Input: part model. Units: mm. Frame: model coordinates. Face numbers are marked on the shaded views. A direction names the side the tool comes from. Round coordinates to 2 decimals unless told otherwise and drop trailing zeros. Order: outer loops, then holes, each group sorted by start corner. A loop starts at its lowest first (then second) coordinate and runs counter-clockwise, first axis right, second up.
Item 1: Reachability of the marked faces 1 and 2 from +Z, -Z, +X, -X, +Y, -Y: full face, straight path, thin tool, end or side. Return the list, or none.
Item 2: Cut plane B-B on x = 7.5. Output: boundary loops of the cut face in (y, z).
Item 3: Cut plane D-D on z = 8. Give the number of separate pieces and of enclosed holes in the cut face, then the cut area to 3 significant figures.
Item 4: Mould query, pull axis X, two halves, no side actions, for the marked faces 3, 4, 5 and 6. Classes: released by +X, released by -X, zero draft, split by the parting line, or undercut.
Item 5: Line query: L1, parallel to X at y = 32, z = 8; L2, parallel to X at y = -19, z = 6; L3, parallel to Y at x = 36, z = 8.25. Output: solid intervals per line, ascending.
Item 6: Cut plane C-C on y = -7.5. Output: boundary loops of the cut face in (x, z).
Item 7: Cut plane A-A on y = 9. Output: boundary loops of the cut face in (x, z).
Item 8: First-contact query: pin 1 (1.5 mm diameter, centred on x = 3.5, y = -14, fed in from +Z); pin 2 (4.5 mm diameter, centred on x = 29.12, z = 8, fed in from +Y). Flat tips, straight axial feed; report the tip coordinate or a pass-through.
```python
from build123d import *

# Parameters (mm, degrees)
BOSS_EXTRU_1_DEPTH        = 13
COQUE1_T                  = -5
COQUE1_THICKNESS_2_FACE_W = 65
COQUE1_THICKNESS_2_FACE_H = 65
COQUE1_THICKNESS_2_DEPTH  = 2
ENL_V_MAT_EXTRU_1_REACH   = 88.587
ESQUISSE2_R               = 2.5
ENL_V_MAT_EXTRU_2_REACH   = 95.396
ESQUISSE3_R               = 2.5
ESQUISSE4_W               = 15
ESQUISSE4_H               = 15
BOSS_EXTRU_2_DEPTH        = 10
ESQUISSE5_R               = 11.5
ENL_V_MAT_EXTRU_3_DEPTH   = 13


with BuildPart() as part:
    # Esquisse1 → Boss.-Extru.1 (new body)
    with BuildSketch(Plane.XY):
        Polygon((44.118436308, 33.728448276), (54.118436308, 33.728448276), (54.118436308, 23.728448276), (54.118436308, -41.271551724), (-20.881563692, -41.271551724), (-20.881563692, 33.728448276), align=None)
    extrude(amount=BOSS_EXTRU_1_DEPTH)

    # Coque1
    coque1_openings = [part.faces().sort_by_distance(p)[0] for p in [
        (16.618436308, -3.771551724, 13),
    ]]
    offset(amount=COQUE1_T, openings=coque1_openings, kind=Kind.INTERSECTION)

    # Coque1 thickness 2 face (on inner face of the shell) → Coque1 thickness 2 (cut)
    with BuildSketch(Plane(origin=(16.618436308, -3.771551724, 5), x_dir=(-1, 0, 0), z_dir=(0, 0, -1))):
        Rectangle(COQUE1_THICKNESS_2_FACE_W, COQUE1_THICKNESS_2_FACE_H)
    extrude(amount=COQUE1_THICKNESS_2_DEPTH, mode=Mode.SUBTRACT)

    # Enlèv. mat.-Extru.1: up to this face of the body (flat: up to its plane)
    enl_v_mat_extru_1_end = Plane(part.part.faces().sort_by_distance((54.118436308, -3.771551724, 6.5))[0])
    # Esquisse2 → Enlèv. mat.-Extru.1 (cut, up to the picked face)
    with BuildSketch(Plane.ZY.offset(20.881563692), mode=Mode.PRIVATE) as enl_v_mat_extru_1_sk1:
        with Locations(Location((8, -16.271551724, 0), (0, 0, 270))):
            Circle(ESQUISSE2_R)
    enl_v_mat_extru_1_tool1 = split(extrude(enl_v_mat_extru_1_sk1.sketch, amount=-ENL_V_MAT_EXTRU_1_REACH, mode=Mode.PRIVATE), bisect_by=enl_v_mat_extru_1_end, keep=Keep.BOTH, mode=Mode.PRIVATE)
    # Esquisse2 → Enlèv. mat.-Extru.1 (cut, up to the picked face)
    with BuildSketch(Plane.ZY.offset(20.881563692), mode=Mode.PRIVATE) as enl_v_mat_extru_1_sk2:
        with Locations(Location((8, 8.728448276, 0), (0, 0, 270))):
            Circle(ESQUISSE2_R)
    enl_v_mat_extru_1_tool2 = split(extrude(enl_v_mat_extru_1_sk2.sketch, amount=-ENL_V_MAT_EXTRU_1_REACH, mode=Mode.PRIVATE), bisect_by=enl_v_mat_extru_1_end, keep=Keep.BOTH, mode=Mode.PRIVATE)
    add(enl_v_mat_extru_1_tool1.solids().sort_by(Axis((-20.881564, -16.271552, 8), (1, 0, 0)))[0], mode=Mode.SUBTRACT)
    add(enl_v_mat_extru_1_tool2.solids().sort_by(Axis((-20.881564, 8.728448, 8), (1, 0, 0)))[0], mode=Mode.SUBTRACT)

    # Enlèv. mat.-Extru.2: up to this face of the body (flat: up to its plane)
    enl_v_mat_extru_2_end = Plane(part.part.faces().sort_by_distance((16.618436308, 33.728448276, 6.5))[0])
    # Esquisse3 → Enlèv. mat.-Extru.2 (cut, up to the picked face)
    with BuildSketch(Plane.XZ.offset(41.271551724), mode=Mode.PRIVATE) as enl_v_mat_extru_2_sk1:
        with Locations(Location((4.118436308, 8, 0), (0, 0, 270))):
            Circle(ESQUISSE3_R)
    enl_v_mat_extru_2_tool1 = split(extrude(enl_v_mat_extru_2_sk1.sketch, amount=-ENL_V_MAT_EXTRU_2_REACH, mode=Mode.PRIVATE), bisect_by=enl_v_mat_extru_2_end, keep=Keep.BOTH, mode=Mode.PRIVATE)
    # Esquisse3 → Enlèv. mat.-Extru.2 (cut, up to the picked face)
    with BuildSketch(Plane.XZ.offset(41.271551724), mode=Mode.PRIVATE) as enl_v_mat_extru_2_sk2:
        with Locations(Location((29.118436308, 8, 0), (0, 0, 270))):
            Circle(ESQUISSE3_R)
    enl_v_mat_extru_2_tool2 = split(extrude(enl_v_mat_extru_2_sk2.sketch, amount=-ENL_V_MAT_EXTRU_2_REACH, mode=Mode.PRIVATE), bisect_by=enl_v_mat_extru_2_end, keep=Keep.BOTH, mode=Mode.PRIVATE)
    add(enl_v_mat_extru_2_tool1.solids().sort_by(Axis((4.118436, -41.271552, 8), (0, 1, 0)))[0], mode=Mode.SUBTRACT)
    add(enl_v_mat_extru_2_tool2.solids().sort_by(Axis((29.118436, -41.271552, 8), (0, 1, 0)))[0], mode=Mode.SUBTRACT)

    # Esquisse4 → Boss.-Extru.2 (add)
    with BuildSketch(Plane.XY.offset(3)):
        Polygon((-5.881563692, 28.728448276), (-15.881563692, 18.728448276), (-15.881563692, 28.728448276), align=None)
        Polygon((49.118436308, 28.728448276), (49.118436308, 18.728448276), (39.118436308, 28.728448276), align=None)
        Polygon((49.118436308, -36.271551724), (49.118436308, -26.271551724), (39.118436308, -36.271551724), align=None)
        with Locations((-13.381563692, -33.771551724)):
            Rectangle(ESQUISSE4_W, ESQUISSE4_H)
    extrude(amount=BOSS_EXTRU_2_DEPTH)

    # Esquisse5 → Enlèv. mat.-Extru.3 (cut)
    with BuildSketch(Plane.XY.offset(13)):
        with Locations((-20.881563692, -41.271551724)):
            Circle(ESQUISSE5_R)
    extrude(amount=-ENL_V_MAT_EXTRU_3_DEPTH, mode=Mode.SUBTRACT)


solid = part.part
```
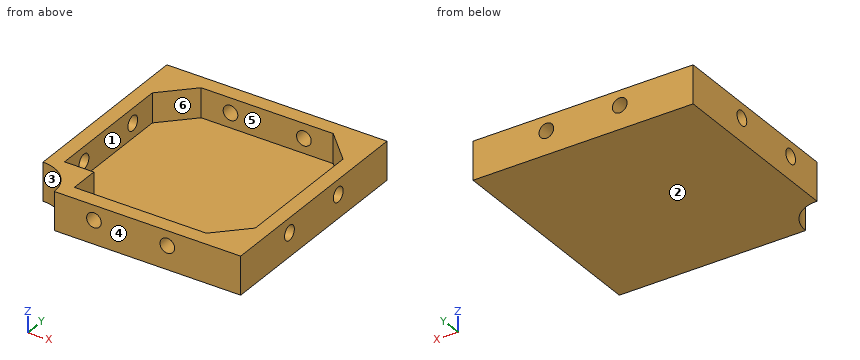
From the geometry:
1. face 1: +Z
1. face 2: -Z, +X, -X, +Y, -Y
2. outline: (-41.27, 0) - (33.73, 0) - (33.73, 13) - (28.73, 13) - (28.73, 3) - (-36.27, 3) - (-36.27, 13) - (-41.27, 13) - close
3. separate pieces: 8
3. enclosed holes: 0
3. area: 1,350 mm2
4. face 3: released by -X
4. face 4: zero draft
4. face 5: undercut
4. face 6: undercut
5. L1: x = -20.88 to 1.62, 6.62 to 26.62, 31.62 to 54.12
5. L2: x = -20.88 to -15.88, 49.12 to 54.12
5. L3: y = -41.27 to -36.27, 28.73 to 33.73
6. outline: (-20.88, 0) - (54.12, 0) - (54.12, 13) - (49.12, 13) - (49.12, 3) - (-15.88, 3) - (-15.88, 13) - (-20.88, 13) - close
7. outline: (-20.88, 0) - (54.12, 0) - (54.12, 5.51) - (49.12, 5.51) - (49.12, 3) - (-15.88, 3) - (-15.88, 5.51) - (-20.88, 5.51) - close; (-20.88, 10.49) - (-15.88, 10.49) - (-15.88, 13) - (-20.88, 13) - close; (49.12, 10.49) - (54.12, 10.49) - (54.12, 13) - (49.12, 13) - close
8. pin 1: stops at z = 3
8. pin 2: passes through
